```python
from build123d import *

# Parameters (mm, degrees)
SKETCH1_W                      = 75
SKETCH1_H                      = 50
BOSS_EXTRUDE1_DEPTH            = 5
CUT_EXTRUDE1_REACH             = 48.165
SKETCH2_R                      = 13
CHAMFER1_SIZE                  = 5
CBORE_FOR_M5_SHCS1_D           = 5.3
CBORE_FOR_M5_SHCS1_CBORE_D     = 9.5
CBORE_FOR_M5_SHCS1_CBORE_DEPTH = 5
CIRPATTERN1_COUNT              = 8
CBORE_FOR_M6_SHCS1_D           = 6.4
CBORE_FOR_M6_SHCS1_CBORE_D     = 11
CBORE_FOR_M6_SHCS1_CBORE_DEPTH = 6
CHAMFER2_SIZE                  = 5
CUT_EXTRUDE2_DEPTH             = 10


with BuildPart() as part:
    # Sketch1 → Boss-Extrude1 (new, symmetric)
    with BuildSketch(Plane(origin=(0, 0, 0), x_dir=(1, 0, 0), z_dir=(0, 1, 0))):
        Rectangle(SKETCH1_W, SKETCH1_H)
    extrude(amount=BOSS_EXTRUDE1_DEPTH, both=True)

    # Sketch2 → Cut-Extrude1 (cut, up to next)
    with BuildSketch(Plane(origin=(0, 5, 0), x_dir=(1, 0, 0), z_dir=(0, 1, 0)), mode=Mode.PRIVATE) as cut_extrude1_sk1:
        with Locations(Location((0, 0, 0), (0, 0, 270))):
            Circle(SKETCH2_R)
    cut_extrude1_tool1 = extrude(cut_extrude1_sk1.sketch, amount=-CUT_EXTRUDE1_REACH, mode=Mode.PRIVATE) & part.part
    add(cut_extrude1_tool1.solids().sort_by_distance((0, 5, 0))[0], mode=Mode.SUBTRACT)

    # Chamfer1
    chamfer1_edges = [part.edges().sort_by_distance(p)[0] for p in [
        (0, 5, -13),
    ]]
    chamfer(chamfer1_edges, length=CHAMFER1_SIZE)

    # CBORE for M5 SHCS1 (through all)
    with Locations(Plane(origin=(0, 5, 0), x_dir=(1, 0, 0), z_dir=(0, 1, 0))):
        with Locations((-6.696960066, 16.167891819)):
            cbore_for_m5_shcs1 = CounterBoreHole(CBORE_FOR_M5_SHCS1_D / 2, CBORE_FOR_M5_SHCS1_CBORE_D / 2, CBORE_FOR_M5_SHCS1_CBORE_DEPTH)

    # CirPattern1: CBORE for M5 SHCS1 ×8 about axis
    cirpattern1_axis = Axis((0, 0, 0), (0, 1, 0))
    for i in range(1, CIRPATTERN1_COUNT):
        add(cbore_for_m5_shcs1.rotate(cirpattern1_axis, i * 360 / CIRPATTERN1_COUNT), mode=Mode.SUBTRACT)

    # CBORE for M6 SHCS1 (through all)
    with Locations(Plane(origin=(0, -5, 0), x_dir=(-1, 0, 0), z_dir=(0, -1, 0))):
        with Locations((30, -17.5), (30, 17.5)):
            CounterBoreHole(CBORE_FOR_M6_SHCS1_D / 2, CBORE_FOR_M6_SHCS1_CBORE_D / 2, CBORE_FOR_M6_SHCS1_CBORE_DEPTH)

    # Chamfer2
    chamfer2_edges = [part.edges().sort_by_distance(p)[0] for p in [
        (-37.5, 0, 25),
        (-37.5, 0, -25),
    ]]
    chamfer(chamfer2_edges, length=CHAMFER2_SIZE)

    # Sketch10 → Cut-Extrude2 (cut)
    with BuildSketch(Plane(origin=(0, 5, 0), x_dir=(1, 0, 0), z_dir=(0, 1, 0))):
        with BuildLine():
            ThreePointArc((0, 25), (17.67766953, 17.67766953), (25, 0))
            ThreePointArc((25, 0), (17.677669539, -17.67766952), (2.6e-08, -25))
            Line((2.6e-08, -25), (37.5, -25))
            Line((37.5, -25), (37.5, 25))
            Line((37.5, 25), (0, 25))
        make_face()
    extrude(amount=-CUT_EXTRUDE2_DEPTH, mode=Mode.SUBTRACT)


solid = part.part
```
Geometry: final body of the model. Coordinates: model frame, mm. A direction names the side the tool comes from. Coordinates: 2 decimals unless noted, no trailing zeros. Order: outer loops, then holes, each group sorted by start corner. A loop starts at its lowest first (then second) coordinate and runs counter-clockwise, first axis right, second up. Notation, with made-up numbers: (55.25, -24.5) - (114.25, -24.5) arc R21 ccw to (114.25, 2.5) - close; hole circle Ø9 at (74.25, 55.25). An arc over 180 degrees is marked (long way). Return JSON: item names as keys, results as strings. Group by question number.
1. Set-up query: faces 1 (the face through (-32.4, 1, -15.1)), 2 (the face through (15.153, -2.535, -9.145)), 3 (the face through (7, 0, -13)). Return all of +Z, -Z, +X, -X, +Y, -Y with unobstructed straight access to the full face (end or side cutting, diameter ignored); none if empty.
2. Cut plane B-B (y = -0.75). Count the separate pieces of the cut face and the enclosed holes in it, plus the area to 3 significant figures.
3. Pull-direction query (X, two-part tool) for faces 4 (the face through (-35, 0.1, -22.5)), 5 (the face through (9.145, -2.535, 15.153)), 6 (the face through (-16, 0, 25)); classes: pulls with the +X half, pulls with the -X half, needs draft (parallel to the pull), parting line crosses it, or undercut.
4. Pin query (flat end, axial travel): pin 1 (5 mm diameter, centred on x = 6.5, y = 1.5, fed in from +Z); pin 2 (23.5 mm diameter, centred on x = 0, z = 0, fed in from +Y); pin 3 (7.5 mm diameter, centred on x = -6.5, z = 16, fed in from +Y). Return the tip coordinate at first contact, or that it passes through.
5. Cut plane A-A (x = -30). Output: boundary loops of the cut face in (y, z).
6. Material intervals for line 1 along Z through (x, y) = (-30, -1.75); line 2 along Z through (x, y) = (18, 4.5); line 3 along X through (y, z) = (-3.75, -8), sorted ascending. Write a range as [from, to].
7. Cut plane C-C (y = 3). Output: boundary loops of the cut face in (x, z).
Resolved:
{
 "1": {"face 1": "-Y", "face 2": "+Y, -Y", "face 3": "+Y"},
 "2": {"separate pieces": "1", "enclosed holes": "11", "area": "1,930 mm²"},
 "3": {"face 4": "pulls with the -X half", "face 5": "undercut", "face 6": "needs draft"},
 "4": {"pin 1": "stops at z = 24.68", "pin 2": "passes through", "pin 3": "stops at y = 0"},
 "5": {"outline": "(-5, -25) - (5, -25) - (5, -20.7) - (1, -20.7) - (1, -23) - (-5, -23) - close; (-5, -12) - (1, -12) - (1, -14.3) - (5, -14.3) - (5, 14.3) - (1, 14.3) - (1, 12) - (-5, 12) - close; (-5, 23) - (1, 23) - (1, 20.7) - (5, 20.7) - (5, 25) - (-5, 25) - close"},
 "6": {"line 1": "z = [-25, -23], [-12, 12], [23, 25]", "line 2": "z = [-17.35, -11.08], [-2.31, 2.31], [11.08, 17.35]", "line 3": "x = [-37.5, -18.48], [-13.86, -10.25], [10.25, 13.86], [18.48, 23.69]"},
 "7": {"outline": "(-37.5, -20) - (-32.5, -25) - (0, -25) arc R25 ccw to (0, 25) - (-32.5, 25) - (-37.5, 20) - close; hole circle Ø6.4 at (-30, -17.5); hole circle Ø6.4 at (-30, 17.5); hole (-15.88, -1.96) arc R4.75 ccw (long way) to (-12.61, -9.85) arc R16 ccw to (-9.85, -12.61) arc R4.75 ccw (long way) to (-1.96, -15.88) arc R16 ccw to (1.96, -15.88) arc R4.75 ccw (long way) to (9.85, -12.61) arc R16 ccw to (12.61, -9.85) arc R4.75 ccw (long way) to (15.88, -1.96) arc R16 ccw to (15.88, 1.96) arc R4.75 ccw (long way) to (12.61, 9.85) arc R16 ccw to (9.85, 12.61) arc R4.75 ccw (long way) to (1.96, 15.88) arc R16 ccw to (-1.96, 15.88) arc R4.75 ccw (long way) to (-9.85, 12.61) arc R16 ccw to (-12.61, 9.85) arc R4.75 ccw (long way) to (-15.88, 1.96) arc R16 ccw to start"}
}
